from build123d import *

# Parameters (mm, degrees)
F0_R     = 1.7145
F1_DEPTH = 9.7028
F2_DEPTH = 18.923
F3_F1_R  = 0.381
F3_F2_R  = 0.381
F4_W     = 9.144
F4_H     = 9.144
F5_DEPTH = 25.4
F6_SIZE  = 1.27
F8_DEPTH = 25.4
F4_W_2   = 15.24
F4_H_2   = 15.24
F4_W_3   = 12.192
F4_H_3   = 12.192
F9_DEPTH = 6.35
F10_R    = 2.54


with BuildPart() as f1:
    # F0 (on Top) → F1 (new body)
    with BuildSketch(Plane.XY):
        with BuildLine():
            ThreePointArc((-9.7536, 0), (0, -9.7536), (9.7536, 0))
            ThreePointArc((9.7536, 0), (0, 9.7536), (-9.7536, 0))
        make_face()
        Circle(F0_R, mode=Mode.SUBTRACT)
    extrude(amount=F1_DEPTH)

    # F0 (on Top) → F2 (join)
    with BuildSketch(Plane.XY):
        with BuildLine():
            Line((9.7536, -15.24), (9.7536, 0))
            ThreePointArc((9.7536, 0), (0, -9.7536), (-9.7536, 0))
            Line((-9.7536, 0), (-9.7536, -15.24))
            Line((-9.7536, -15.24), (9.7536, -15.24))
        make_face()
    extrude(amount=F2_DEPTH)

    # F3: fillet of radius 0.381 on 3 edges, made by hand

    # F3_f1
    f3_f1_edges = [f1.edges().sort_by_distance(p)[0] for p in [
        (9.7536, 0, 14.3129),
    ]]
    fillet(f3_f1_edges, radius=F3_F1_R)

    # F3_f2
    f3_f2_edges = [f1.edges().sort_by_distance(p)[0] for p in [
        (-9.7536, 0, 14.3129),
    ]]
    fillet(f3_f2_edges, radius=F3_F2_R)

    # F4 (on face) → F5 (join)
    with BuildSketch(Plane.XZ.offset(15.24)):
        with Locations((0, 9.500099346)):
            Rectangle(F4_W, F4_H)
    extrude(amount=F5_DEPTH)

    # F6
    f6_edges = [f1.edges().sort_by_distance(p)[0] for p in [
        (0, -40.64, 4.928099),
        (4.572, -40.64, 9.500099),
        (0, -40.64, 14.072099),
        (-4.572, -40.64, 9.500099),
    ]]
    chamfer(f6_edges, length=F6_SIZE)

    # F8 (cut): a face of the model
    f8_faces = [f1.faces().sort_by_distance(p)[0] for p in [
        (0, -40.64, 9.500099346),
    ]]
    extrude(f8_faces, amount=-F8_DEPTH, mode=Mode.SUBTRACT)

    # F4 (on face) → F9 (cut)
    with BuildSketch(Plane.XZ.offset(15.24)):
        with Locations((0, 9.500099346)):
            Rectangle(F4_W_2, F4_H_2)
        with Locations((0, 9.500099346)):
            Rectangle(F4_W_3, F4_H_3, mode=Mode.SUBTRACT)
    extrude(amount=-F9_DEPTH, mode=Mode.SUBTRACT)

    # F10
    f10_edges = [f1.edges().sort_by_distance(p)[0] for p in [
        (0, 9.7536, 0),
        (9.7536, -7.62, 0),
        (-9.7536, -7.62, 0),
    ]]
    fillet(f10_edges, radius=F10_R)


solid = f1.part
Can you work these out from the model? Positions are in its coordinate system, mm. A direction names the side the tool comes from. Coordinates: 2 decimals unless noted, no trailing zeros. Write each loop counter-clockwise with the first axis right and the second up, starting at its lowest first coordinate (ties: lowest second). Pieces come first, ordered by that corner, then holes. Notation, with made-up numbers: (65, -36.75) -> (80, -36.75) arc R16 ccw to (80, -21.75) -> close; hole circle Ø5 at (43, 54). An arc over 180 degrees is marked (long way). Write each question's results on one line, items separated by ' | '. Start each with the question number.
Q1. Imagine slicing it at B-B (x = 0). Write out the boundary of the cut face in (y, z), then the cut area to 3 significant figures.
Q2. I'm going to push flat-ended pins straight in: pin 1 (10 mm diameter, centred on x = -2, y = -4, fed in from +Z); pin 2 (6 mm diameter, centred on y = -19, z = 5.5, fed in from -X); pin 3 (3.5 mm diameter, centred on x = 1.5, z = 8.5, fed in from -Y); pin 4 (5 mm diameter, centred on y = -17, z = 6.5, fed in from -X). Where does each tip first touch, or does it pass through?
Q3. On a 3-axis mill with a long thin cutter (end or side, diameter ignored), from which of +Z, -Z, +X, -X, +Y, -Y can I reach the whole of each face in a straight line? I mean faces 4 (the face through (0, -12, 3.404)), 5 (the face through (-0.06, -40.01, 13.43)), 6 (the face through (2, 0, 9.703)), 7 (the face through (-9.029, -7.727, 0.764)), 8 (the face through (0, -27, 4.928)). Say none if no direction works.
Q4. We'd pull the mould along X, two halves only. Please class faces 1 (the face through (9.754, -8, 11)), 2 (the face through (0, -15.24, 18)), 3 (the face through (0, -12, 15.596)): +X half, -X half, draft (parallel to the pull), parting line (faces both ways), or undercut.
Q5. Imagine slicing it at C-C (z = 7.5). Write out the boundary of the cut face in (x, y).
Q6. If I drill on probe 1 along Z at (x, y) = (-5.5, -11); probe 2 along X at (y, z) = (-24.5, 6.5); probe 3 along Y at (x, z) = (0, 4.75), over which ranges is the centre line in solid material (lowest first)?
Q7. Imagine slicing it at A-A (y = -10.5). Write out the boundary of the cut face in (x, z).
Taken from the geometry:
1) outline: (-40.64, 6.2) -> (-39.37, 4.93) -> (-15.24, 4.93) -> (-15.24, 3.4) -> (-8.89, 3.4) -> (-8.89, 1.88) -> (-15.24, 1.88) -> (-15.24, 0) -> (-1.71, 0) -> (-1.71, 9.7) -> (-9.75, 9.7) -> (-9.75, 15.6) -> (-15.24, 15.6) -> (-15.24, 14.07) -> (-39.37, 14.07) -> (-40.64, 12.8) -> (-15.24, 12.8) -> (-15.24, 6.2) -> close; (-15.24, 17.12) -> (-9.75, 17.12) -> (-9.75, 18.92) -> (-15.24, 18.92) -> close; (1.71, 0) -> (7.21, 0) arc R2.54 ccw to (9.75, 2.54) -> (9.75, 9.7) -> (1.71, 9.7) -> close | area: 303 mm^2
2) pin 1: stops at z = 9.7 | pin 2: stops at x = -4.57 | pin 3: stops at y = -15.24 | pin 4: stops at x = -9.75
3) face 4: -Y | face 5: +Z, +X, -X, -Y | face 6: +Z, +Y | face 7: -Z, -X, +Y, -Y | face 8: -Z, +X, -X, -Y
4) face 1: +X half | face 2: draft | face 3: undercut
5) outline: (-9.75, -15.24) -> (-7.62, -15.24) -> (-7.62, -8.89) -> (-6.1, -8.89) -> (-6.1, -15.24) -> (-4.57, -15.24) -> (-4.57, -39.37) -> (-3.3, -40.64) -> (-3.3, -15.24) -> (3.3, -15.24) -> (3.3, -40.64) -> (4.57, -39.37) -> (4.57, -15.24) -> (6.1, -15.24) -> (6.1, -8.89) -> (7.62, -8.89) -> (7.62, -15.24) -> (9.75, -15.24) -> (9.75, 0) arc R9.75 ccw to (-9.75, 0) -> close; hole circle Ø3.43 at (0, 0)
6) probe 1: z = 0 to 1.88, 3.4 to 15.6, 17.12 to 18.92 | probe 2: x = -4.57 to -3.3, 3.3 to 4.57 | probe 3: y = -15.24 to -1.71, 1.71 to 9.75
7) outline: (-9.75, 2.54) arc R2.54 ccw to (-7.21, 0) -> (7.21, 0) arc R2.54 ccw to (9.75, 2.54) -> (9.75, 18.92) -> (-9.75, 18.92) -> close; (-6.1, 3.4) -> (6.1, 3.4) -> (6.1, 15.6) -> (-6.1, 15.6) -> close; hole (-7.62, 1.88) -> (7.62, 1.88) -> (7.62, 17.12) -> (-7.62, 17.12) -> close
